Build history of the part. All positions in model axes, mm. A direction names the side the tool comes from. Round coordinates to 2 decimals unless told otherwise and drop trailing zeros. Write item = value, one per line.
from build123d import *

# Parameters (mm, degrees)
F0_R     = 17.884061545
F1_DEPTH = 1
F2_R     = 17.884061545
F2_R_2   = 15.884061545
F3_DEPTH = 120
F5_DEPTH = 100
F6_R     = 2
F7_DEPTH = 121.0010007


with BuildPart() as f1:
    # F0 (on Top) → F1 (new body)
    with BuildSketch(Plane.XY):
        Circle(F0_R)
    extrude(amount=F1_DEPTH)

    # F2 (on face) → F3 (join)
    with BuildSketch(Plane(origin=(0, 0, 0), x_dir=(1, 0, 0), z_dir=(0, 0, -1))):
        Circle(F2_R)
        Circle(F2_R_2, mode=Mode.SUBTRACT)
    extrude(amount=F3_DEPTH)

    # F4 (on Right) → F5 (cut, symmetric)
    with BuildSketch(Plane.YZ):
        with BuildLine():
            add(Edge.make_bspline(
                [(-23.545185104, -2.931100782), (-12.2797633222, -3.5261581086), (11.4767752963, -34.9586093489), (12.414609837, -94.1865478451), (15.1815395802, -125.3380775452)],
                knots=[0, 0, 0, 0, 0.3949910862, 1, 1, 1, 1], degree=3))
            Line((-23.545185104, -2.931100782), (-23.545185104, -130.5240243673))
            Line((-23.545185104, -130.5240243673), (15.1815395802, -125.3380775452))
        make_face()
    extrude(amount=F5_DEPTH, both=True, mode=Mode.SUBTRACT)

    # F6 (on face) → F7 (cut, through all)
    with BuildSketch(Plane.XY.offset(1)):
        with Locations((-6.0105, 6.0103152788)):
            Circle(F6_R)
        with Locations((6.0105, 6.0103152788)):
            Circle(F6_R)
        with Locations((6.0105, -6.0103152788)):
            Circle(F6_R)
        with Locations((-6.0105, -6.0103152788)):
            Circle(F6_R)
    extrude(amount=-F7_DEPTH, mode=Mode.SUBTRACT)


solid = f1.part
1. Tool access for faces 1 (the face through (0, 0, 0)), 2 (the face through (-4.94, -4.32, 0.51)): list every direction of +Z, -Z, +X, -X, +Y, -Y with a clear straight run to the whole face (end or side of a thin tool).
Responses:
face_1 = -Z
face_2 = +Z, -Z
2. Mould opens along Y. For faces 3 (the face through (0, 0, 1)), 4 (the face through (-3.88, 17.46, -45.21)), 5 (the face through (-5.088, 4.236, 0.507)), 6 (the face through (-3.443, 15.506, -45.827)) say: pulls with the +Y half, pulls with the -Y half, needs draft (parallel to the pull), parting line crosses it, or undercut.
Responses:
face_3 = needs draft
face_4 = parting line crosses it
face_5 = undercut
face_6 = undercut
3. Probe probe 1 along Z at (x, y) = (-12.5, 5); probe 2 along Y at (x, z) = (0, -26.5); probe 3 along X at (y, z) = (12, -32.5). List the from-to ranges inside material, lowest first.
Responses:
probe_1 = 0 to 1
probe_2 = 15.88 to 17.88
probe_3 = -13.26 to -10.41, 10.41 to 13.26
4. Flat gauge pins, fed straight in: pin 1 (6 mm diameter, centred on x = 2.5, z = -46.5, fed in from -Y); pin 2 (1 mm diameter, centred on y = 5.5, z = -27.5, fed in from -X); pin 3 (2 mm diameter, centred on x = 13.5, z = -15.5, fed in from -Y). Where does each tip first touch, or does it go through?
Responses:
pin_1 = 14.9
pin_2 = -17.17
pin_3 = 6.48
